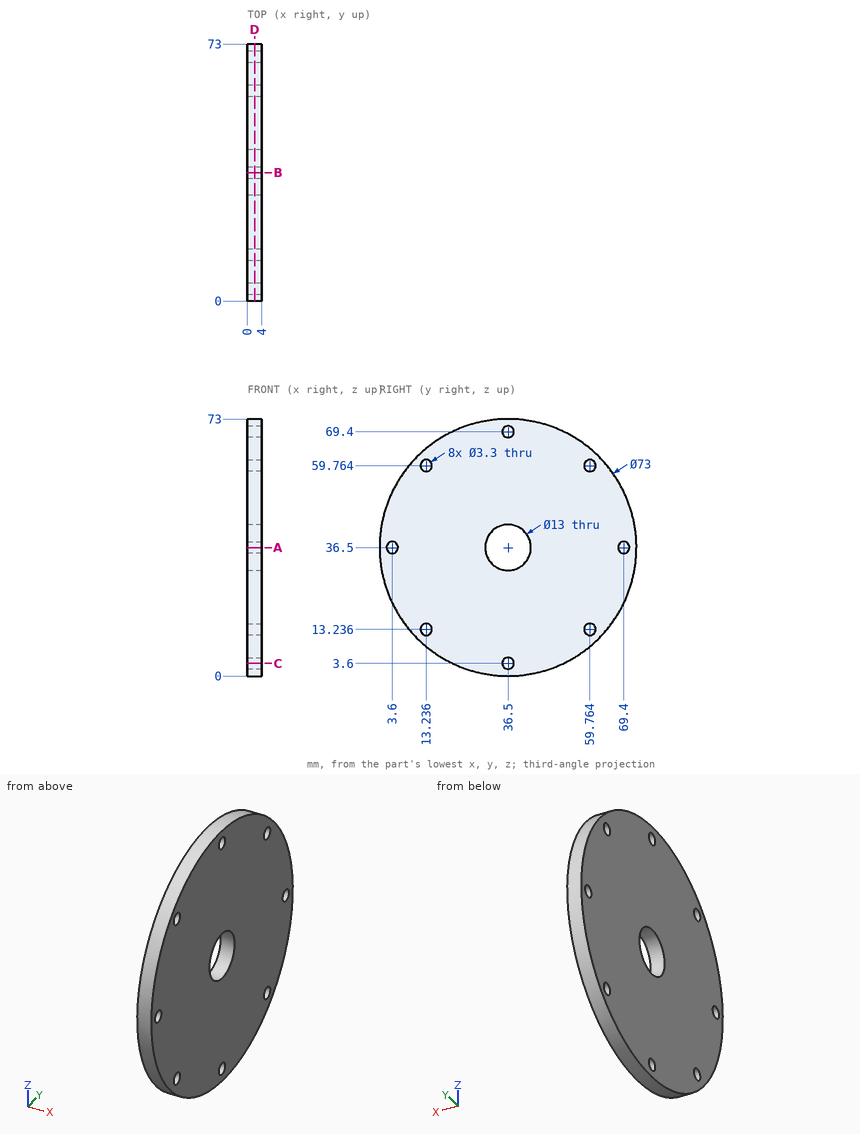
Part print with two shaded views. Sizes in mm from the minimum x, y, z corner. Coordinates: 2 decimals unless noted, no trailing zeros. Order: outer loops, then holes, each group sorted by start corner. A loop starts at its lowest first (then second) coordinate and runs counter-clockwise, first axis right, second up.
(1) Saw through at C-C, the plane z = 3.6. Write the cut outline in (x, y), and give its area (3 significant figures).
Solution:
outline: (0, 20.69) - (4, 20.69) - (4, 34.85) - (0, 34.85) - close; (0, 38.15) - (4, 38.15) - (4, 52.31) - (0, 52.31) - close
area: 113 mm2
(2) Drill centre lines: L1, parallel to Y at x = 0.95, z = 36.5; L2, parallel to Z at x = 2.7, y = 68.5; L3, parallel to Y at x = 2.65, z = 5. Where is each one in solid material? Low to high.
Solution:
L1: y = 0 to 1.95, 5.25 to 30, 43 to 67.75, 71.05 to 73
L2: z = 18.94 to 35.12, 37.88 to 54.06
L3: y = 18.06 to 35.63, 37.37 to 54.94
(3) Pin check, flat tips, straight feed: pin 1 Ø1.5 at (x, y) = (1, 61) entering from -Z; pin 2 Ø1.5 at (x, z) = (1.5, 7.5) entering from -Y. Stop position of each tip, or through.
Solution:
pin 1: stops at z = 8.78
pin 2: stops at y = 13.39
(4) Saw through at A-A, the plane z = 36.5. Write the cut outline in (x, y), and give its area (3 significant figures).
Solution:
outline: (0, 0) - (4, 0) - (4, 1.95) - (0, 1.95) - close; (0, 5.25) - (4, 5.25) - (4, 30) - (0, 30) - close; (0, 43) - (4, 43) - (4, 67.75) - (0, 67.75) - close; (0, 71.05) - (4, 71.05) - (4, 73) - (0, 73) - close
area: 214 mm2
(5) Saw through at D-D, the plane x = 2.05. Count the separate pieces of the cut face and the enclosed holes in it, and give its area (3 significant figures).
Solution:
separate pieces: 1
enclosed holes: 9
area: 3,980 mm2
